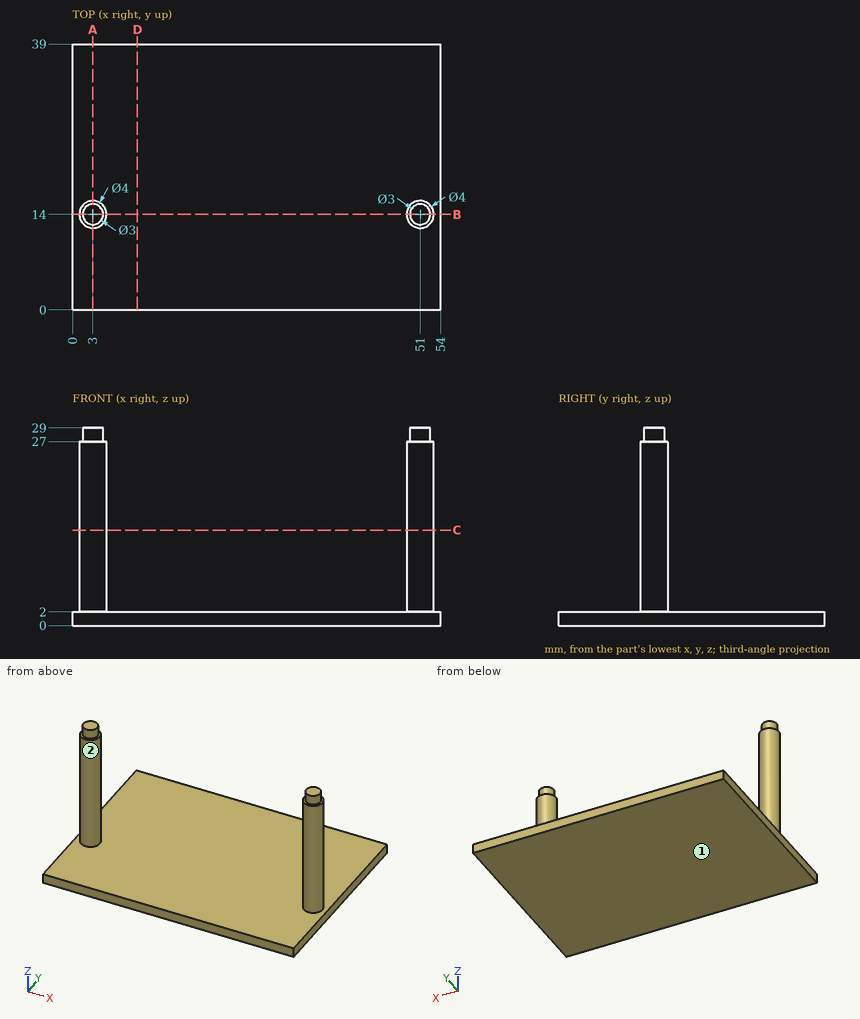
Source: three-view drawing plus pictorial views. Frame: mm from the lowest corner of the part. Round coordinates to 2 decimals unless told otherwise and drop trailing zeros. Loops run counter-clockwise (first coordinate to the right, second up) from the corner with the lowest first, then second, coordinate; pieces in that order, holes last.
Item 1: Line query: L1, parallel to Z at x = 50, y = 3.5; L2, parallel to Y at x = 51, z = 6.5; L3, parallel to Y at x = 49.5, z = 23.25. Output: solid intervals per line, ascending.
Checked values:
L1: z = 0 to 2
L2: y = 12 to 16
L3: y = 12.68 to 15.32
Item 2: Mould query, pull axis X, two halves, no side actions, for the marked faces 1 and 2. Classes: released by +X, released by -X, zero draft, split by the parting line, or undercut.
Checked values:
face 1: zero draft
face 2: undercut
Item 3: Section A-A, the plane x = 3. Output: boundary loops of the cut face in (y, z).
Checked values:
outline: (0, 0) - (39, 0) - (39, 2) - (16, 2) - (16, 27) - (15.5, 27) - (15.5, 29) - (12.5, 29) - (12.5, 27) - (12, 27) - (12, 2) - (0, 2) - close
Item 4: Section C-C, the plane z = 14. Output: boundary loops of the cut face in (x, y).
Checked values:
outline: circle Ø4 at (3, 14); circle Ø4 at (51, 14)
Item 5: Section D-D, the plane x = 9.5. Output: boundary loops of the cut face in (y, z).
Checked values:
outline: (0, 0) - (39, 0) - (39, 2) - (0, 2) - close
Item 6: Section B-B, the plane y = 14. Output: boundary loops of the cut face in (x, z), plus the area to 3 significant figures.
Checked values:
outline: (0, 0) - (54, 0) - (54, 2) - (53, 2) - (53, 27) - (52.5, 27) - (52.5, 29) - (49.5, 29) - (49.5, 27) - (49, 27) - (49, 2) - (5, 2) - (5, 27) - (4.5, 27) - (4.5, 29) - (1.5, 29) - (1.5, 27) - (1, 27) - (1, 2) - (0, 2) - close
area: 320 mm2
Item 7: Contact query for flat-ended pins moving along their axis: P1, Ø1.5, axis at x = 23.5, y = 9.5, coming from the +Z side; P2, Ø6, axis at x = 44, z = 19, coming from the -Y side. Output: stop coordinate, or through.
Checked values:
P1: stops at z = 2
P2: passes through
